```python
from build123d import *

# Parameters (mm, degrees)
F1_DEPTH = 17.5
F2_SIZE  = 2
F3_W     = 42
F3_H     = 69
F4_DEPTH = 15


with BuildPart() as f1:
    # F0 (on Top) → F1 (new body)
    with BuildSketch(Plane.XY):
        Polygon((112.5, 63), (0, 63), (-112.5, 63), (-112.5, 0), (-112.5, -63), (0, -63), (112.5, -63), (112.5, 0), align=None)
    extrude(amount=F1_DEPTH)

    # F2
    f2_edges = [f1.edges().sort_by_distance(p)[0] for p in [
        (-112.5, 0, 0),
        (0, -63, 0),
        (112.5, 0, 0),
        (0, 63, 0),
        (-112.5, -63, 8.75),
        (112.5, -63, 8.75),
        (112.5, 63, 8.75),
        (-112.5, 63, 8.75),
    ]]
    chamfer(f2_edges, length=F2_SIZE)

    # F3 (on face) → F4 (cut)
    with BuildSketch(Plane.XY.offset(17.5)):
        with Locations((89, 26.5)):
            Rectangle(F3_W, F3_H)
        with Locations((44.5, 26.5)):
            Rectangle(F3_W, F3_H)
        with Locations((0, 26.5)):
            Rectangle(F3_W, F3_H)
        with Locations((-44.5, 26.5)):
            Rectangle(F3_W, F3_H)
        with Locations((-89, 26.5)):
            Rectangle(F3_W, F3_H)
    extrude(amount=-F4_DEPTH, mode=Mode.SUBTRACT)


solid = f1.part
```
The listing builds one solid part. Answer for the finished solid, in the listing's coordinates (mm). Round coordinates to 2 decimals unless told otherwise and drop trailing zeros. Write each loop counter-clockwise with the first axis right and the second up, starting at its lowest first coordinate (ties: lowest second). Pieces come first, ordered by that corner, then holes. Notation, with made-up numbers: (82, 47.5) -> (102, 47.5) arc R24 ccw to (102, 69.5) -> close; hole circle Ø1 at (72, 17). An arc over 180 degrees is marked (long way). Use CSV: the item, a comma, the result in double quotes. Start each with the question number.
(1) Section C-C on y = 24.5 is taken. Give the vertices of the cut face in (x, z), then the cut area to 4 significant figures.
(2) Section B-B on x = -98 is taken. Give the vertices of the cut face in (y, z), then the cut area to 3 significant figures.
(3) The mould has two halves that part along X. Classify faces 1 (the face through (-112.5, 1, 10)), 2 (the face through (-45, -8, 10)), 3 (the face through (-89, 61, 10)), 4 (the face through (-2, 1, 0)): released by +X, released by -X, zero draft, split by the parting line, or undercut.
(4) This flat-tipped pin is pushed along its axis until it touches: pin 1 (12.5 mm diameter, centred on x = 37.5, y = 21, fed in from +Z). Where does it stop, or does it pass through?
(5) Section A-A on z = 9 is taken. Give the vertices of the cut face in (x, y), then the cut area to 3 significant figures.
(6) Consider L1, parallel to X at y = 31, z = 10.75; L2, parallel to Y at x = 54.5, z = 13.75; L3, parallel to Z at x = 62, y = 30. Determine where each line is inside the solid, lowest interval first. Write a range as from..to.
A:
1,outline,"(-112.5, 2) -> (-110.5, 0) -> (110.5, 0) -> (112.5, 2) -> (112.5, 17.5) -> (110, 17.5) -> (110, 2.5) -> (68, 2.5) -> (68, 17.5) -> (65.5, 17.5) -> (65.5, 2.5) -> (23.5, 2.5) -> (23.5, 17.5) -> (21, 17.5) -> (21, 2.5) -> (-21, 2.5) -> (-21, 17.5) -> (-23.5, 17.5) -> (-23.5, 2.5) -> (-65.5, 2.5) -> (-65.5, 17.5) -> (-68, 17.5) -> (-68, 2.5) -> (-110, 2.5) -> (-110, 17.5) -> (-112.5, 17.5) -> close"
1,area,"783.5 mm²"
2,outline,"(-63, 2) -> (-61, 0) -> (61, 0) -> (63, 2) -> (63, 17.5) -> (61, 17.5) -> (61, 2.5) -> (-8, 2.5) -> (-8, 17.5) -> (-63, 17.5) -> close"
2,area,"1,170 mm²"
3,face 1,"released by -X"
3,face 2,"undercut"
3,face 3,"undercut"
3,face 4,"zero draft"
4,pin 1,"stops at z = 2.5"
5,outline,"(-112.5, -61) -> (-110.5, -63) -> (110.5, -63) -> (112.5, -61) -> (112.5, 61) -> (110.5, 63) -> (-110.5, 63) -> (-112.5, 61) -> close; hole (-110, -8) -> (-68, -8) -> (-68, 61) -> (-110, 61) -> close; hole (-65.5, -8) -> (-23.5, -8) -> (-23.5, 61) -> (-65.5, 61) -> close; hole (-21, -8) -> (21, -8) -> (21, 61) -> (-21, 61) -> close; hole (23.5, -8) -> (65.5, -8) -> (65.5, 61) -> (23.5, 61) -> close; hole (68, -8) -> (110, -8) -> (110, 61) -> (68, 61) -> close"
5,area,"13,900 mm²"
6,L1,"x = -112.5..-110, -68..-65.5, -23.5..-21, 21..23.5, 65.5..68, 110..112.5"
6,L2,"y = -63..-8, 61..63"
6,L3,"z = 0..2.5"
